Verification items for this drawing (mm, ordinates from the low corner). A direction names the side the tool comes from. Round coordinates to 2 decimals unless told otherwise and drop trailing zeros. Order: outer loops, then holes, each group sorted by start corner. A loop starts at its lowest first (then second) coordinate and runs counter-clockwise, first axis right, second up. Notation, with made-up numbers: (77.25, 71.5) -> (81.25, 71.5) arc R34 ccw to (81.25, 109.5) -> close; hole circle Ø5 at (-12.75, -6). An arc over 180 degrees is marked (long way). Return JSON: item names as keys, results as strings. Group by question number.
Item 1: Scan lines: probe 1 along X at (y, z) = (24.55, 50.8); probe 2 along Y at (x, z) = (17, 17.5); probe 3 along X at (y, z) = (12.5, 62). Record each from-to range of solid material in increasing order. Write a range as from..to.
Item 2: Draft check along Y on the marked faces 1, 2, 3 and 4. Enter one of: pulls with the +Y half, pulls with the -Y half, needs draft (parallel to the pull), parting line crosses it, or undercut.
Item 3: Sectioned sample at A-A on z = 50.8. Record the cut outline in (x, y).
Item 4: Access from +Z, -Z, +X, -X, +Y, -Y to the whole of each face (thin tool, end or side, straight path). Record for the marked faces 5 and 6.
Item 5: Sectioned sample at D-D on z = 84. Record the cut outline in (x, y).
Item 6: Sectioned sample at C-C on x = 38. Record the cut outline in (y, z), plus the area to 3 significant figures.
Item 7: Sectioned sample at B-B on y = 6.5. Record the cut outline in (x, z), plus the area to 3 significant figures.
Item 8: Depth check by flat-ended pin: pin 1 Ø3 at (x, z) = (31.75, 63.5) entering from -Y. Enter the tip coordinate at first touch or a pass-through.
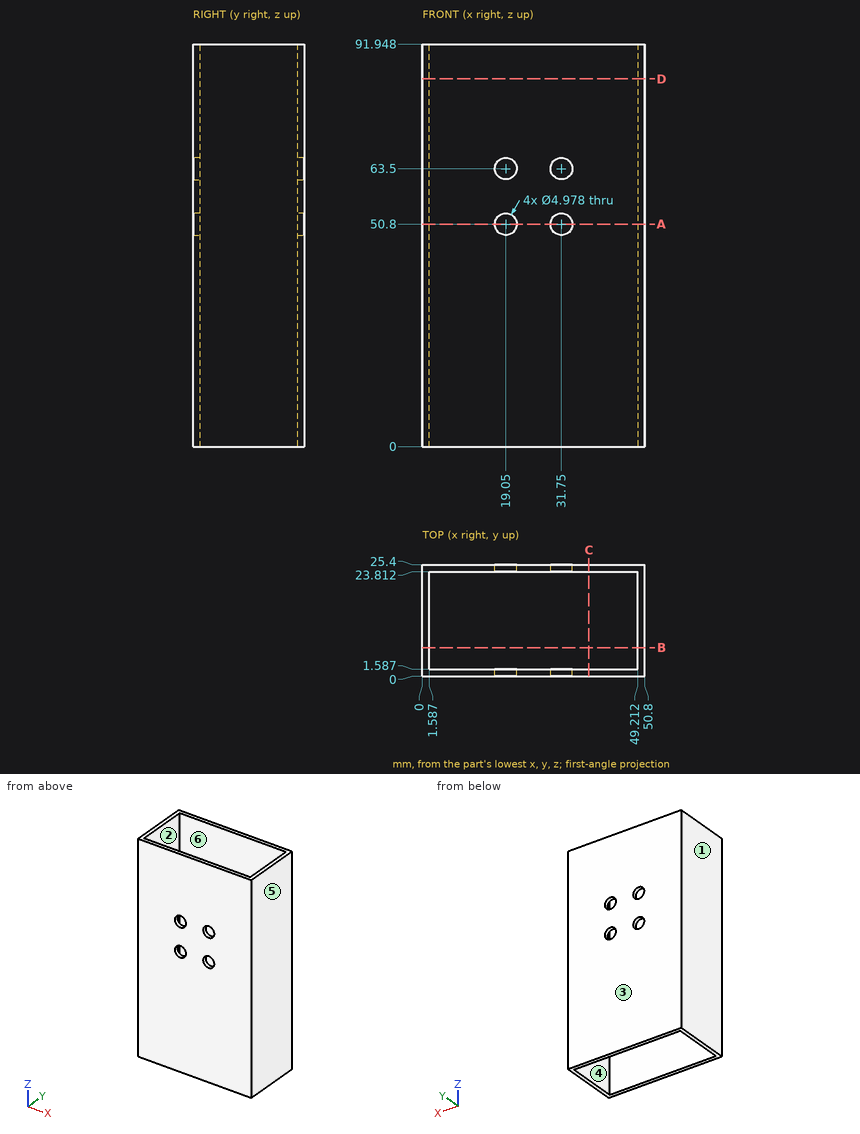
Recorded:
{
 "1": {"probe 1": "0..16.56, 21.54..29.26, 34.24..50.8", "probe 2": "0..1.59, 23.81..25.4", "probe 3": "0..1.59, 49.21..50.8"},
 "2": {"face 1": "needs draft", "face 2": "undercut", "face 3": "pulls with the +Y half", "face 4": "undercut"},
 "3": {"outline": "(0, 0) -> (16.56, 0) -> (16.56, 1.59) -> (1.59, 1.59) -> (1.59, 23.81) -> (16.56, 23.81) -> (16.56, 25.4) -> (0, 25.4) -> close; (21.54, 0) -> (29.26, 0) -> (29.26, 1.59) -> (21.54, 1.59) -> close; (21.54, 23.81) -> (29.26, 23.81) -> (29.26, 25.4) -> (21.54, 25.4) -> close; (34.24, 0) -> (50.8, 0) -> (50.8, 25.4) -> (34.24, 25.4) -> (34.24, 23.81) -> (49.21, 23.81) -> (49.21, 1.59) -> (34.24, 1.59) -> close"},
 "4": {"face 5": "+Z, -Z, +X, +Y, -Y", "face 6": "+Z, -Z"},
 "5": {"outline": "(0, 0) -> (50.8, 0) -> (50.8, 25.4) -> (0, 25.4) -> close; hole (1.59, 1.59) -> (49.21, 1.59) -> (49.21, 23.81) -> (1.59, 23.81) -> close"},
 "6": {"outline": "(0, 0) -> (1.59, 0) -> (1.59, 91.95) -> (0, 91.95) -> close; (23.81, 0) -> (25.4, 0) -> (25.4, 91.95) -> (23.81, 91.95) -> close", "area": "292 mm²"},
 "7": {"outline": "(0, 0) -> (1.59, 0) -> (1.59, 91.95) -> (0, 91.95) -> close; (49.21, 0) -> (50.8, 0) -> (50.8, 91.95) -> (49.21, 91.95) -> close", "area": "292 mm²"},
 "8": {"pin 1": "through"}
}
